```python
from build123d import *

# Parameters (mm, degrees)
BOSS_EXTRUDE1_DEPTH        = 38
SKETCH1_3_W                = 100
SKETCH1_3_H                = 35
SKETCH1_3_W_2              = 70
SKETCH1_3_H_2              = 16
BOSS_EXTRUDE2_DEPTH        = 16
FILLET1_RADIUS             = 19
FILLET1_LENGTH             = 25
F_19_0_19_DIAMETER_HOLE1_D = 19
F_13_0_13_DIAMETER_HOLE1_D = 13


with BuildPart() as part:
    # Sketch1 → Boss-Extrude1 (new body)
    with BuildSketch(Plane(origin=(0, 0, 0), x_dir=(0, 0, -1), z_dir=(1, 0, 0))):
        Polygon((100, 10), (100, 83), (125, 83), (125, 0), (0, 0), (0, 10), align=None)
    extrude(amount=BOSS_EXTRUDE1_DEPTH)

    # Sketch1<3> → Boss-Extrude2 (add)
    with BuildSketch(Plane(origin=(0, 0, 0), x_dir=(0, 0, -1), z_dir=(1, 0, 0))):
        with Locations((50, 27.5)):
            Rectangle(SKETCH1_3_W, SKETCH1_3_H)
        with Locations((51, 27)):
            Rectangle(SKETCH1_3_W_2, SKETCH1_3_H_2, mode=Mode.SUBTRACT)
    extrude(amount=BOSS_EXTRUDE2_DEPTH)

    # Fillet1: full round fillet: the end face becomes a half cylinder, R = half its width
    fillet1_face = Plane((19, 83, -112.5), x_dir=(0, 0, -1), z_dir=(0, 1, 0))  # on the end face: x along it, z out of the body
    fillet1_slab = fillet1_face.offset(-FILLET1_RADIUS / 2) * Box(FILLET1_LENGTH, 2 * FILLET1_RADIUS, FILLET1_RADIUS, mode=Mode.PRIVATE)  # the body's end, R deep
    fillet1_round = Plane((19, 64, -112.5), x_dir=(0, 1, 0), z_dir=(0, 0, -1)) * Cylinder(FILLET1_RADIUS, FILLET1_LENGTH, mode=Mode.PRIVATE)  # its axis R under the face
    add(fillet1_slab - fillet1_round, mode=Mode.SUBTRACT)

    # Ø19.0 (19) Diameter Hole1 (through all)
    with Locations(Plane(origin=(19, 64, -100), x_dir=(1, 0, 0), z_dir=(0, 0, 1))):
        with Locations((0, 0)):
            Hole(F_19_0_19_DIAMETER_HOLE1_D / 2)

    # Ø13.0 (13) Diameter Hole1 (through all)
    with Locations(Plane(origin=(25, 10, -25), x_dir=(0, 0, 1), z_dir=(0, 1, 0))):
        with Locations((0, 0), (-50, 0)):
            Hole(F_13_0_13_DIAMETER_HOLE1_D / 2)


solid = part.part
```
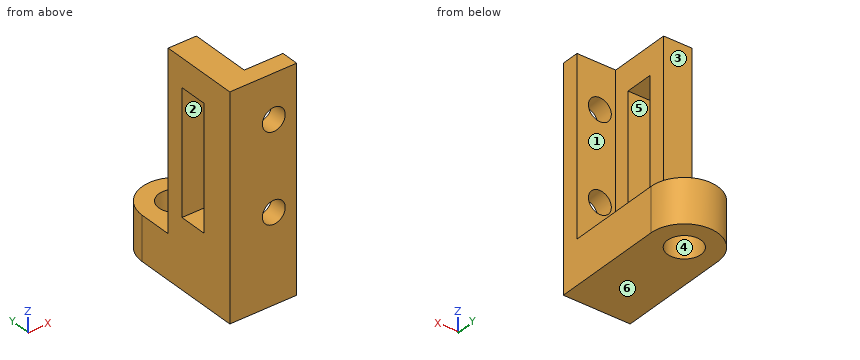
Source: CAD feature listing. Evaluate the final solid. Frame: model axes, mm. Face numbers are marked on the shaded views. A direction names the side the tool comes from. Coordinates: 2 decimals unless noted, no trailing zeros. Loops run counter-clockwise (first coordinate to the right, second up) from the corner with the lowest first, then second, coordinate; pieces in that order, holes last. Notation, with made-up numbers: M 48,-32 L 54,-32 A17 ccw 54,-10 Z; hole C -39,-1 d5. An arc over 180 degrees is marked long. Use a Markdown table: item, result. Add a question column.
Q1. Section query B-B, the plane y = 24. Return loops of the section in (x, z).
Q2. Section query C-C, the plane z = -104. Return loops of the section in (x, y), and give its area (3 significant figures).
Q3. Material intervals for L1, parallel to Y at x = 5, z = -85.5; L2, parallel to Y at x = 19, z = -112.25; L3, parallel to Z at x = 24, y = 9, sorted ascending.
Q4. First-contact query: pin 1 (8 mm diameter, centred on x = 21, z = -73, fed in from -Y); pin 2 (1.5 mm diameter, centred on x = 23, y = 74, fed in from +Z); pin 3 (3 mm diameter, centred on y = 40, z = -75.5, fed in from +X); pin 4 (6 mm diameter, centred on x = 4.5, z = -83.5, fed in from +Y). Flat tips, straight axial feed; report the tip coordinate or a pass-through.
Q5. Access query for the marked faces 1, 2 and 3. Directions: +Z, -Z, +X, -X, +Y, -Y. A direction counts if a zero-diameter tool reaches every point of the face in a straight line with its end or side. Return the directions, or none.
Q6. Draft query along Z for the marked faces 4, 5 and 6. Return one class per face: pulls with the +Z half, pulls with the -Z half, needs draft (parallel to the pull), parting line crosses it, or undercut.
Q7. Section query D-D, the plane x = 6. Return loops of the section in (y, z).
Q8. Section query A-A, the plane z = -43.5. Return loops of the section in (x, y).
Result:
| question | item | result |
|---|---|---|
| 1 | outline | M 0,-125 L 38,-125 L 38,-100 L 16,-100 L 16,-86 L 0,-86 Z; M 0,-16 L 16,-16 L 16,0 L 0,0 Z |
| 2 | outline | M 0,0 L 38,0 L 38,64 A19 ccw 0,64 Z; hole C 19,64 d19 |
| 2 | area | 2,720 mm2 |
| 3 | L1 | y = 0 to 19, 35 to 45 |
| 3 | L2 | y = 0 to 54.5, 73.5 to 83 |
| 3 | L3 | z = -125 to -81.42, -68.58 to -31.42, -18.58 to 0 |
| 4 | pin 1 | stops at y = 0 |
| 4 | pin 2 | stops at z = -100 |
| 4 | pin 3 | stops at x = 16 |
| 4 | pin 4 | stops at y = 45 |
| 5 | face 1 | +Z, +X, +Y |
| 5 | face 2 | +X, -X |
| 5 | face 3 | +Z, +X, -X, +Y |
| 6 | face 4 | needs draft |
| 6 | face 5 | undercut |
| 6 | face 6 | pulls with the -Z half |
| 7 | outline | M 0,-125 L 77.86,-125 L 77.86,-100 L 45,-100 L 45,0 L 0,0 Z; hole M 19,-86 L 35,-86 L 35,-16 L 19,-16 Z |
| 8 | outline | M 0,0 L 38,0 L 38,10 L 16,10 L 16,19 L 0,19 Z; M 0,35 L 16,35 L 16,45 L 0,45 Z |
